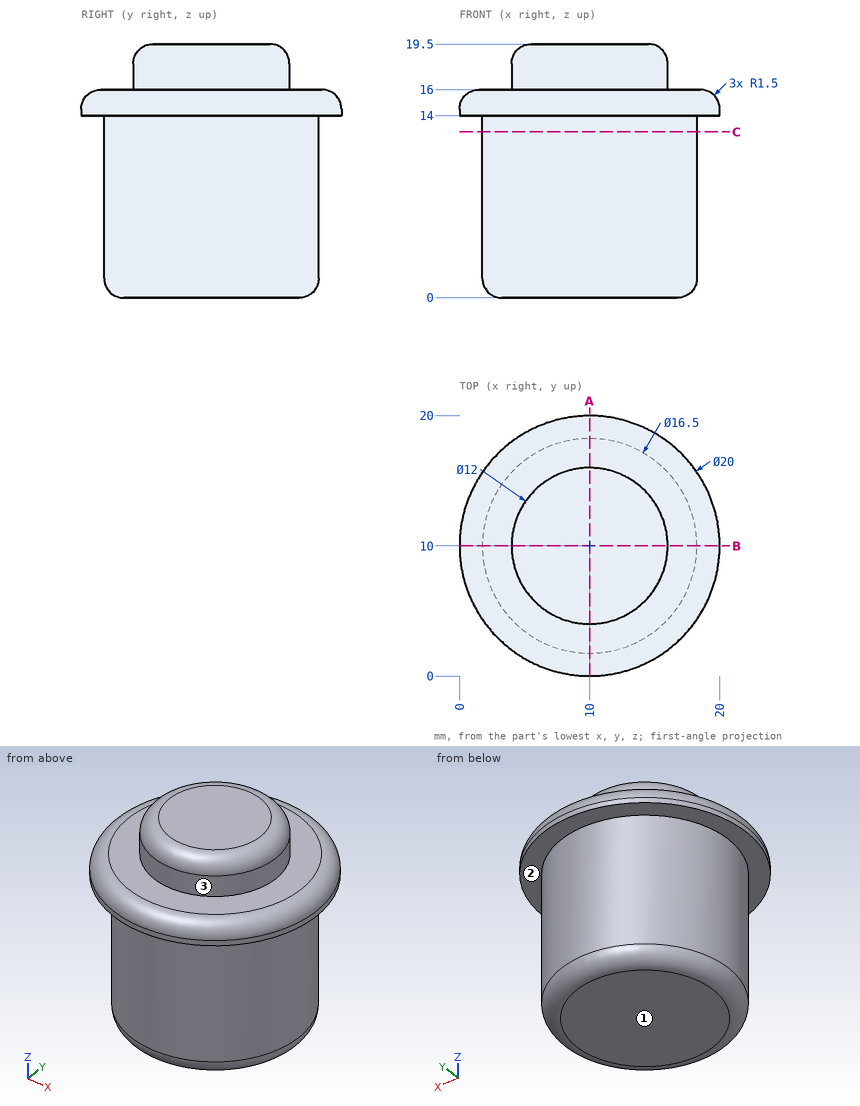
Answer from the drawing. Dimensions are ordinates in mm from the lowest x, y and z of the part. A direction names the side the tool comes from. Coordinates: 2 decimals unless noted, no trailing zeros. Loops run counter-clockwise (first coordinate to the right, second up) from the corner with the lowest first, then second, coordinate; pieces in that order, holes last.
1) Consider probe 1 along Z at (x, y) = (5.5, 3); probe 2 along X at (y, z) = (9.75, 3.25); probe 3 along Y at (x, z) = (5.25, 1.5). Determine where each line is inside the solid, lowest interval first.
Results:
probe 1: z = 14 to 16
probe 2: x = 1.75 to 18.25
probe 3: y = 3.25 to 16.75
2) Section A-A (x = 10) is taken. Give the vertices of the cut face in (y, z).
Results:
outline: (0, 14) - (1.75, 14) - (1.75, 1.5) arc R1.5 ccw to (3.25, 0) - (16.75, 0) arc R1.5 ccw to (18.25, 1.5) - (18.25, 14) - (20, 14) - (20, 14.5) arc R1.5 ccw to (18.5, 16) - (16, 16) - (16, 18) arc R1.5 ccw to (14.5, 19.5) - (5.5, 19.5) arc R1.5 ccw to (4, 18) - (4, 16) - (1.5, 16) arc R1.5 ccw to (0, 14.5) - close
3) Section C-C (z = 12.75) is taken. Give the vertices of the cut face in (x, y).
Results:
outline: circle Ø16.5 at (10, 10)
4) Flat-ended cylindrical pins translate along their axes: pin 1 (4 mm diameter, centred on x = 14.5, z = 6.5, fed in from -Y); pin 2 (1 mm diameter, centred on y = 10, z = 8, fed in from -X); pin 3 (2 mm diameter, centred on x = 4.5, y = 11, fed in from +Z). Find the tip coordinate at first contact, or state that the pin passes through.
Results:
pin 1: stops at y = 2.14
pin 2: stops at x = 1.75
pin 3: stops at z = 19.5
5) For the marked faces 1, 2 and 3, determine the directions among +Z, -Z, +X, -X, +Y, -Y from which every point of the face is accessible in a straight line to the end or side of a thin tool.
Results:
face 1: -Z, +X, -X, +Y, -Y
face 2: -Z
face 3: +Z
